The model under review builds one solid part; all positions refer to its coordinate system, in mm. Face numbers are marked on the shaded views. A direction names the side the tool comes from. Round coordinates to 2 decimals unless told otherwise and drop trailing zeros. Write each loop counter-clockwise with the first axis right and the second up, starting at its lowest first coordinate (ties: lowest second). Pieces come first, ordered by that corner, then holes. Notation, with made-up numbers: (-38.75, 73.5) - (-0.75, 73.5) arc R22 cw to (-0.75, 112.5) - close; hole circle Ø10 at (54, 40). An arc over 180 degrees is marked (long way). Return JSON: item names as keys, results as strings.
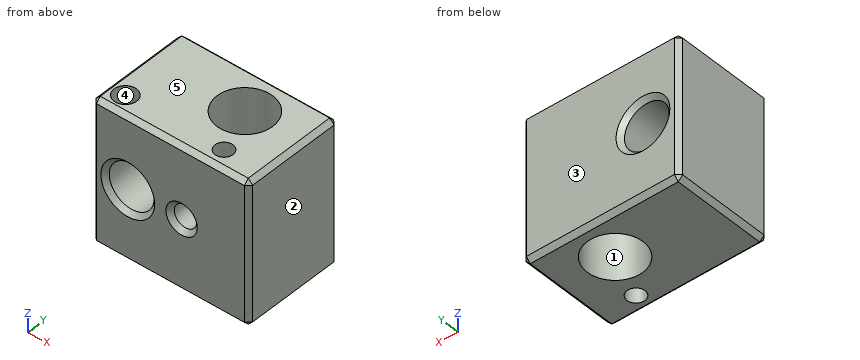
from build123d import *

# Parameters (mm, degrees)
SKETCH1_W                       = 17.5
SKETCH1_H                       = 16
BOSS_EXTRUDE1_DEPTH             = 11.5
SKETCH2_R                       = 3.1
SKETCH2_R_2                     = 1
CUT_EXTRUDE1_DEPTH              = 17
F_2_5_2_5_DIAMETER_HOLE1_D      = 2.5
F_2_5_2_5_DIAMETER_HOLE1_DEPTH  = 4.5
TAP_DRILL_FOR_M6X1_0_TAP1_D     = 5
TAP_DRILL_FOR_M3X0_5_TAP1_D     = 2.5
TAP_DRILL_FOR_M3X0_5_TAP1_DEPTH = 6.999
TAP_DRILL_FOR_M3X0_5_TAP1_TIP   = 0.751075774
CHAMFER1_SIZE                   = 0.5


with BuildPart() as part:
    # Sketch1 → Boss-Extrude1 (new body)
    with BuildSketch(Plane(origin=(0, 0, 0), x_dir=(1, 0, 0), z_dir=(0, 1, 0))):
        Rectangle(SKETCH1_W, SKETCH1_H)
    extrude(amount=BOSS_EXTRUDE1_DEPTH)

    # Sketch2 → Cut-Extrude1 (cut, through all)
    with BuildSketch(Plane.XY.offset(8)):
        with Locations((2.25, 7)):
            Circle(SKETCH2_R)
        with Locations((4.25, 2)):
            Circle(SKETCH2_R_2)
    extrude(amount=-CUT_EXTRUDE1_DEPTH, mode=Mode.SUBTRACT)

    # Ø2.5 (2.5) Diameter Hole1
    with Locations(Plane.XY.offset(8)):
        with Locations((-6.75, 2)):
            Hole(F_2_5_2_5_DIAMETER_HOLE1_D / 2, depth=F_2_5_2_5_DIAMETER_HOLE1_DEPTH)

    # Tap Drill for M6x1.0 Tap1 (through all)
    with Locations(Plane(origin=(0, 11.5, 0), x_dir=(1, 0, 0), z_dir=(0, 1, 0))):
        with Locations((-4.75, 0)):
            Hole(TAP_DRILL_FOR_M6X1_0_TAP1_D / 2)

    # Tap Drill for M3x0.5 Tap1
    with Locations(Plane(origin=(0, 0, 0), x_dir=(-1, 0, 0), z_dir=(0, -1, 0))):
        with Locations((-1.25, 0)):
            Hole(TAP_DRILL_FOR_M3X0_5_TAP1_D / 2, depth=TAP_DRILL_FOR_M3X0_5_TAP1_DEPTH)
            with Locations((0, 0, -(TAP_DRILL_FOR_M3X0_5_TAP1_DEPTH + TAP_DRILL_FOR_M3X0_5_TAP1_TIP / 2))):  # 118° drill point
                Cone(0, TAP_DRILL_FOR_M3X0_5_TAP1_D / 2, TAP_DRILL_FOR_M3X0_5_TAP1_TIP, mode=Mode.SUBTRACT)

    # Chamfer1
    chamfer1_edges = [part.edges().sort_by_distance(p)[0] for p in [
        (0, 11.5, -8),
        (-8.75, 11.5, 0),
        (-2.25, 11.5, 0),
        (-2.25, 0, 0),
        (0, 0, 0),
        (0, 11.5, 8),
        (-8.75, 0, 0),
        (0, 0, -8),
        (8.75, 0, 0),
        (0, 0, 8),
        (8.75, 11.5, 0),
        (-8.75, 5.75, 8),
        (-8.75, 5.75, -8),
        (8.75, 5.75, -8),
        (8.75, 5.75, 8),
    ]]
    chamfer(chamfer1_edges, length=CHAMFER1_SIZE)


solid = part.part
(1) Add section C-C (y = 1.5). Write out the cut boundary in (x, z), plus the area to 3 significant figures.
Filled in:
{"outline": "(-8.75, -7.5) - (-8.25, -8) - (3.38, -8) - (3.38, 8) - (-5.6, 8) - (-5.6, 3.5) - (-7.9, 3.5) - (-7.9, 8) - (-8.25, 8) - (-8.75, 7.5) - close; (5.12, -8) - (8.25, -8) - (8.75, -7.5) - (8.75, 7.5) - (8.25, 8) - (5.12, 8) - close; hole circle Ø5 at (-4.75, 0); hole circle Ø2.5 at (1.25, 0)", "area": "217 mm2"}
(2) Add section B-B (z = 5.75). Write out the cut boundary in (x, y).
Filled in:
{"outline": "(-8.75, 0.5) - (-8.25, 0) - (8.25, 0) - (8.75, 0.5) - (8.75, 11) - (8.25, 11.5) - (-8.25, 11.5) - (-8.75, 11) - close; hole circle Ø2.5 at (-6.75, 2); hole circle Ø6.2 at (2.25, 7); hole circle Ø2 at (4.25, 2)"}
(3) For the marked faces 4 and 5, list the 3-axis set-ups (+Z, -Z, +X, -X, +Y, -Y) from which the entire face can be reached by the end or side of a thin tool; tool diameter is ignored.
Filled in:
{"face 4": "+Z", "face 5": "+Z, +X, -X, +Y, -Y"}
(4) Add section A-A (x = -4.75). Write out the cut boundary in (y, z).
Filled in:
{"outline": "(0, -7.5) - (0.5, -8) - (11, -8) - (11.5, -7.5) - (11.5, -3) - (11, -2.5) - (0.5, -2.5) - (0, -3) - close; (0, 3) - (0.5, 2.5) - (11, 2.5) - (11.5, 3) - (11.5, 7.5) - (11, 8) - (0.5, 8) - (0, 7.5) - close"}
(5) Mouldability with a two-part tool opening along Y and no side actions: class the marked faces 1, 2 and 3 as released by +Y, released by -Y, zero draft, split by the parting line, or undercut.
Filled in:
{"face 1": "undercut", "face 2": "zero draft", "face 3": "released by +Y"}
(6) Add section D-D (y = 7.25). Write out the cut boundary in (x, z), plus the area to 3 significant figures.
Filled in:
{"outline": "(-8.75, -7.5) - (-8.25, -8) - (-0.84, -8) - (-0.84, 8) - (-8.25, 8) - (-8.75, 7.5) - close; (5.34, -8) - (8.25, -8) - (8.75, -7.5) - (8.75, 7.5) - (8.25, 8) - (5.34, 8) - close; hole circle Ø5 at (-4.75, 0)", "area": "161 mm2"}
(7) Wall thickness on line 1 (X direction, y = 3.65, z = 0); line 2 (X direction, y = 1.25, z = 7); line 3 (Y direction, x = 3.5, z = 4.25): over which ranges is each line inside the solid? List them lowest first.
Filled in:
{"line 1": "x = -8.75 to -7.25, -2.25 to 0, 2.5 to 8.75", "line 2": "x = -8.75 to -7.75, -5.75 to 3.59, 4.91 to 8.75", "line 3": "y = 0 to 1.34, 2.66 to 4.16, 9.84 to 11.5"}
